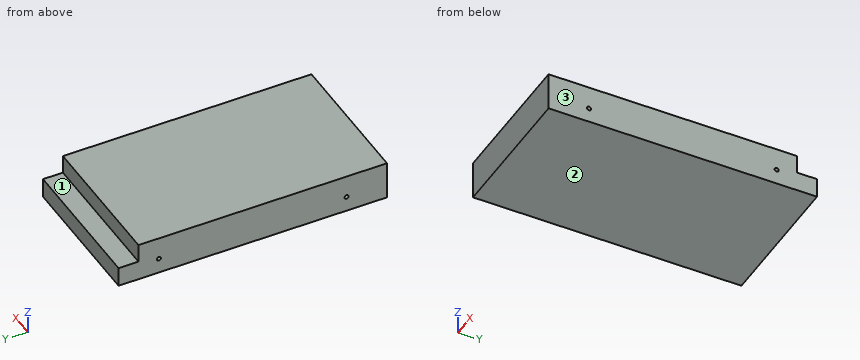
from build123d import *

# Parameters (mm, degrees)
F0_W      = 115
F0_H      = 216
F1_DEPTH  = 31
F3_W      = 115
F3_H      = 16
F4_DEPTH  = 15
F6_R      = 1.65
F7_DEPTH  = 5
F9_R      = 1.65
F10_DEPTH = 5


with BuildPart() as f1:
    # F0 (on Top) → F1 (new body)
    with BuildSketch(Plane.XY):
        Rectangle(F0_W, F0_H)
    extrude(amount=F1_DEPTH)

    # F3 (on offset) → F4 (cut)
    with BuildSketch(Plane.XY.offset(31)):
        with Locations((0, 100)):
            Rectangle(F3_W, F3_H)
    extrude(amount=-F4_DEPTH, mode=Mode.SUBTRACT)

    # F6 (on offset) → F7 (cut)
    with BuildSketch(Plane.YZ.offset(57.5)):
        with Locations((-75.5, 12)):
            Circle(F6_R)
        with Locations((75.5, 12.5)):
            Circle(F6_R)
    extrude(amount=-F7_DEPTH, mode=Mode.SUBTRACT)

    # F9 (on offset) → F10 (cut)
    with BuildSketch(Plane(origin=(-57.5, 0, 0), x_dir=(0, -1, 0), z_dir=(-1, 0, 0))):
        with Locations((75.5, 12.5)):
            Circle(F9_R)
        with Locations((-75.5, 12.5)):
            Circle(F9_R)
    extrude(amount=-F10_DEPTH, mode=Mode.SUBTRACT)


solid = f1.part
Can you work these out from the model? Positions are in its coordinate system, mm. Face numbers are marked on the shaded views. Coordinates: 2 decimals unless noted, no trailing zeros. Write each loop counter-clockwise with the first axis right and the second up, starting at its lowest first coordinate (ties: lowest second). Pieces come first, ordered by that corner, then holes. Notation, with made-up numbers: (32.5, 23) - (91.5, 23) arc R12 ccw to (91.5, 34) - close; hole circle Ø11 at (55.5, 78). An arc over 180 degrees is marked (long way). Return JSON: item names as keys, results as strings. Group by question number.
Item 1: I'm going to push flat-ended pins straight in: pin 1 Ø7.5 at (x, z) = (6.5, 26.5) entering from +Y; pin 2 Ø2.5 at (y, z) = (-75.5, 12) entering from +X; pin 3 Ø2 at (y, z) = (75.5, 12.5) entering from -X. Where does each tip first touch, or does it pass through?
Item 2: Please list where these lines run through material, in increasing order: probe 1 along Z at (x, y) = (53.8, 75.5); probe 2 along Y at (x, z) = (21.5, 25).
Item 3: If we section it at A-A (x = -14.5): Write out the boundary of the cut face in (y, z).
Item 4: We'd pull the mould along Z, two halves only. Please class the marked faces 1, 2 and 3: pulls with the +Z half, pulls with the -Z half, needs draft (parallel to the pull), parting line crosses it, or undercut.
Item 5: If we section it at B-B (z = 19): Write out the boundary of the cut face in (x, y).
Return value:
{
 "1": {"pin 1": "stops at y = 92", "pin 2": "stops at x = 52.5", "pin 3": "stops at x = -52.5"},
 "2": {"probe 1": "z = 0 to 10.85, 14.15 to 31", "probe 2": "y = -108 to 92"},
 "3": {"outline": "(-108, 0) - (108, 0) - (108, 16) - (92, 16) - (92, 31) - (-108, 31) - close"},
 "4": {"face 1": "pulls with the +Z half", "face 2": "pulls with the -Z half", "face 3": "needs draft"},
 "5": {"outline": "(-57.5, -108) - (57.5, -108) - (57.5, 92) - (-57.5, 92) - close"}
}
